For this review, take the finished solid that the model builds, in its own axes (mm). A direction names the side the tool comes from. Give positions to 0.01 mm unless a question says otherwise; leave off trailing zeros. Write each loop counter-clockwise with the first axis right and the second up, starting at its lowest first coordinate (ties: lowest second). Pieces come first, ordered by that corner, then holes. Notation, with made-up numbers: (33.5, 61) -> (40.5, 61) arc R19 ccw to (40.5, 95) -> close; hole circle Ø2 at (56.5, 24). An arc over 180 degrees is marked (long way). Return JSON: item names as keys, results as strings.
from build123d import *

# Parameters (mm, degrees)
CYLINDER003_R     = 3
CYLINDER003_DEPTH = 5
BOX006_W          = 22
BOX006_H          = 5
BOX006_DEPTH      = 21
BOX007_W          = 10
BOX007_H          = 12
BOX007_DEPTH      = 21
CYLINDER007_R     = 5
CYLINDER007_DEPTH = 8
BOX010_W          = 3
BOX010_H          = 16
BOX010_DEPTH      = 3
CYLINDER006_R     = 8
CYLINDER006_DEPTH = 10
CYLINDER001_R     = 4
CYLINDER001_DEPTH = 84
BOX017_W          = 8
BOX017_H          = 5
BOX017_DEPTH      = 8
BOX018_W          = 8
BOX018_H          = 5
BOX018_DEPTH      = 8
BOX019_W          = 22
BOX019_H          = 84
BOX019_DEPTH      = 5
BOX003_W          = 99
BOX003_H          = 74
BOX003_DEPTH      = 29
BOX002_W          = 104
BOX002_H          = 84
BOX002_DEPTH      = 27


with BuildPart() as pivotmountinghole:
    # Cylinder003 → Cylinder003 (new body)
    with BuildSketch(Plane(origin=(19.5, 28.5, 14), x_dir=(1, 0, 0), z_dir=(0, -1, 0))):
        Circle(CYLINDER003_R)
    extrude(amount=CYLINDER003_DEPTH)


with BuildPart() as pivotplate:
    # Box006 → Box006 (new body)
    with BuildSketch(Plane(origin=(15, 23.5, 8), x_dir=(1, 0, 0), z_dir=(0, 0, 1))):
        with Locations((11, 2.5)):
            Rectangle(BOX006_W, BOX006_H)
    extrude(amount=BOX006_DEPTH)


with BuildPart() as pivotmount:
    # Box007 → Box007 (new body)
    with BuildSketch(Plane(origin=(37, 16.5, 8), x_dir=(1, 0, 0), z_dir=(0, 0, 1))):
        with Locations((5, 6)):
            Rectangle(BOX007_W, BOX007_H)
    extrude(amount=BOX007_DEPTH)

    # Fusion003: union PivotPlate
    add(pivotplate.part)

    # Cut003: cut PivotMountingHole
    add(pivotmountinghole.part, mode=Mode.SUBTRACT)


with BuildPart() as topspringholeinner:
    # Cylinder007 → Cylinder007 (new body)
    with BuildSketch(Plane(origin=(65, 35, 19), x_dir=(1, 0, 0), z_dir=(0, 0, 1))):
        Circle(CYLINDER007_R)
    extrude(amount=CYLINDER007_DEPTH)


with BuildPart() as topspringholecutout:
    # Box010 → Box010 (new body)
    with BuildSketch(Plane(origin=(63.5, 27, 23), x_dir=(1, 0, 0), z_dir=(0, 0, 1))):
        with Locations((1.5, 8)):
            Rectangle(BOX010_W, BOX010_H)
    extrude(amount=BOX010_DEPTH)

    # Fusion005: union TopSpringHoleInner
    add(topspringholeinner.part)


with BuildPart() as topspringcaptive:
    # Cylinder006 → Cylinder006 (new body)
    with BuildSketch(Plane(origin=(65, 35, 19), x_dir=(1, 0, 0), z_dir=(0, 0, 1))):
        Circle(CYLINDER006_R)
    extrude(amount=CYLINDER006_DEPTH)

    # Cut005: cut TopSpringHoleCutout
    add(topspringholecutout.part, mode=Mode.SUBTRACT)


with BuildPart() as pivotaxistop:
    # Cylinder001 → Cylinder001 (new body)
    with BuildSketch(Plane(origin=(19.5, 77, 14), x_dir=(1, 0, 0), z_dir=(0, -1, 0))):
        Circle(CYLINDER001_R)
    extrude(amount=CYLINDER001_DEPTH)


with BuildPart() as obj1:
    # Box017 → Box017 (new body)
    with BuildSketch(Plane(origin=(61, 72, 22), x_dir=(1, 0, 0), z_dir=(0, 0, 1))):
        with Locations((4, 2.5)):
            Rectangle(BOX017_W, BOX017_H)
    extrude(amount=BOX017_DEPTH)


with BuildPart() as obj2:
    # Box018 → Box018 (new body)
    with BuildSketch(Plane(origin=(61, -7, 22), x_dir=(1, 0, 0), z_dir=(0, 0, 1))):
        with Locations((4, 2.5)):
            Rectangle(BOX018_W, BOX018_H)
    extrude(amount=BOX018_DEPTH)


with BuildPart() as toppedalhingecutout:
    # Box019 → Box019 (new body)
    with BuildSketch(Plane(origin=(-7, -7, 29), x_dir=(1, 0, 0), z_dir=(0, 0, 1))):
        with Locations((11, 42)):
            Rectangle(BOX019_W, BOX019_H)
    extrude(amount=BOX019_DEPTH)


with BuildPart() as toppedalcutout:
    # Box003 → Box003 (new body)
    with BuildSketch(Plane(origin=(-7, -2, 0), x_dir=(1, 0, 0), z_dir=(0, 0, 1))):
        with Locations((49.5, 37)):
            Rectangle(BOX003_W, BOX003_H)
    extrude(amount=BOX003_DEPTH)

    # Fusion001: union PivotAxisTop, obj1, obj2, TopPedalHingeCutout
    add(pivotaxistop.part)
    add(obj1.part)
    add(obj2.part)
    add(toppedalhingecutout.part)


with BuildPart() as obj3:
    # Box002 → Box002 (new body)
    with BuildSketch(Plane(origin=(-7, -7, 7), x_dir=(1, 0, 0), z_dir=(0, 0, 1))):
        with Locations((52, 42)):
            Rectangle(BOX002_W, BOX002_H)
    extrude(amount=BOX002_DEPTH)

    # Cut001: cut TopPedalCutout
    add(toppedalcutout.part, mode=Mode.SUBTRACT)

    # Fusion006: union PivotMount, TopSpringCaptive
    add(pivotmount.part)
    add(topspringcaptive.part)


with BuildPart() as obj3_1:
    # Fusion006 placement: moved
    add(obj3.part.moved(Location((-19.5, 0, -14))))


solid = obj3_1.part
1. Add section C-C, the plane x = 31. State the section outline as (y, z) points.
Results found:
{"outline": "(-7, -7) -> (-2, -7) -> (-2, 15) -> (72, 15) -> (72, -7) -> (77, -7) -> (77, 20) -> (-7, 20) -> close"}
2. The part is to be moulded in two halves that separate along Z. For faces 4 (the flat face through (44, 29, 10)), 5 (the flat face through (36, 36, 20)), 6 (the flat face through (17.5, 20, 4)), say which applies: +Z half, -Z half, draft (parallel to the pull), parting line (faces both ways), or undercut.
Results found:
{"face 4": "undercut", "face 5": "+Z half", "face 6": "draft"}
3. Add section D-D, the plane y = 35. State the section outline as (x, z) points.
Results found:
{"outline": "(-4.5, 15) -> (37.5, 15) -> (37.5, 5) -> (40.5, 5) -> (40.5, 13) -> (50.5, 13) -> (50.5, 5) -> (53.5, 5) -> (53.5, 15) -> (72.5, 15) -> (72.5, -7) -> (77.5, -7) -> (77.5, 20) -> (-4.5, 20) -> close"}
4. Add section A-A, the plane z = 0. State the section outline as (x, y) points.
Results found:
{"outline": "(-26.5, -7) -> (-4, -7) -> (-4, -2) -> (-26.5, -2) -> close; (-26.5, 72) -> (-4, 72) -> (-4, 77) -> (-26.5, 77) -> close; (-4.5, 23.5) -> (-3, 23.5) -> (-3, 28.5) -> (-4.5, 28.5) -> close; (3, 23.5) -> (17.5, 23.5) -> (17.5, 16.5) -> (27.5, 16.5) -> (27.5, 28.5) -> (3, 28.5) -> close; (4, -7) -> (77.5, -7) -> (77.5, 77) -> (4, 77) -> (4, 72) -> (72.5, 72) -> (72.5, -2) -> (4, -2) -> close"}
5. Add section B-B, the plane x = 45.5. Count the separate pieces of the cut face and the enclosed holes in it, plus the area to 3 significant figures.
Results found:
{"separate pieces": "5", "enclosed holes": "0", "area": "622 mm²"}
6. For faces 1 (the flat face through (45, -4, 8)), 2 (the cylindrical face through (50.119, 33.085, 8.944)), 3 (the flat face through (49.5, 74, 12)), list the 3-axis set-ups (+Z, -Z, +X, -X, +Y, -Y) from which the entire face can be reached by the end or side of a thin tool; tool diameter is ignored.
Results found:
{"face 1": "-Y", "face 2": "-Z", "face 3": "+Y"}
7. To check wall thickness, follow probe 1 along Y at (x, z) = (-1, 13.5); probe 2 along Y at (x, z) = (26.5, 13.75); probe 3 along Y at (x, z) = (60, 8.25). State the ranges of each line that lie inside material, in increasing order.
Results found:
{"probe 1": "y = -7 to -2, 23.5 to 28.5, 72 to 77", "probe 2": "y = -7 to -2, 16.5 to 28.5, 72 to 77", "probe 3": "y = -7 to -2, 72 to 77"}
8. For pin 1 (1.5 mm diameter, centred on x = -19, y = 75, fed in from +Z); pin 2 (0.5 mm diameter, centred on x = 45.5, z = 15.5, fed in from +Y); pin 3 (0.5 mm diameter, centred on x = 44.5, z = 15.5, fed in from -Y), all flat-tipped, find the tip position at first contact; note any pin that passes through.
Results found:
{"pin 1": "stops at z = 15", "pin 2": "stops at y = 72", "pin 3": "stops at y = -2"}
